The model under review builds one solid part; all positions refer to its coordinate system, in mm. Give positions to 0.01 mm unless a question says otherwise; leave off trailing zeros. Order: outer loops, then holes, each group sorted by start corner. A loop starts at its lowest first (then second) coordinate and runs counter-clockwise, first axis right, second up. Notation, with made-up numbers: (28.25, 77.25) - (32.25, 77.25) arc R16 cw to (32.25, 103.25) - close; hole circle Ø11 at (81, -40). An arc over 180 degrees is marked (long way). Use a Markdown table: item, result. Add a question column.
Autodesk Inventor part; units mm, degrees
ref_plane "YZ Plane" through (0, 0, 0) normal (1, 0, 0) x (0, 1, 0)
ref_plane "XZ Plane" through (0, 0, 0) normal (0, 1, 0) x (-1, 0, 0)
ref_plane "XY Plane" through (0, 0, 0) normal (0, 0, 1) x (1, 0, 0)
sketch "Sketch1" plane through (0, 0, 0) normal (0, 1, 0) x (-1, 0, 0)
  line L0 (169.8625, 0) -> (0, 0)
  line L1 (0, 0) -> (0, -169.8625)
  line L2 (0, -169.8625) -> (25.4, -169.8625)
  line L3 (25.4, -169.8625) -> (25.4, -103.8713)
  line L4 (103.8713, -25.4) -> (169.8625, -25.4)
  line L5 (169.8625, -25.4) -> (169.8625, 0)
  arc A0 (103.8713, -25.4) -> (25.4, -103.8713) centre (66.675, -66.675) ccw
  line L6 (0, 0) -> (66.675, -66.675) construction
  line L7 (0, -20) -> (6.35, -20)
  line L8 (6.35, -20) -> (6.35, -40)
  line L9 (6.35, -40) -> (0, -40)
  line L10 (0, -40) -> (0, -20)
  line L11 (6.35, -60) -> (6.35, -80)
  line L12 (0, -60) -> (6.35, -60)
  line L13 (6.35, -80) -> (0, -80)
  line L14 (6.35, -100) -> (6.35, -120)
  line L15 (0, -100) -> (6.35, -100)
  line L16 (6.35, -120) -> (0, -120)
  line L17 (6.35, -140) -> (6.35, -160)
  line L18 (0, -140) -> (6.35, -140)
  line L19 (6.35, -160) -> (0, -160)
  line L20 (23.368, -27.3469) -> (16.764, -27.3469)
  line L21 (16.764, -27.3469) -> (16.764, -12.0929)
  line L22 (16.764, -12.0929) -> (23.368, -12.0929)
  line L23 (23.368, -12.0929) -> (23.368, -27.3469)
  line L24 (23.368, -27.3469) -> (16.764, -12.0929) construction
  line L25 (16.764, -27.3469) -> (23.368, -12.0929) construction
  line L26 (25.4, -160) -> (16.764, -160)
  line L27 (16.764, -160) -> (16.764, -140)
  line L28 (16.764, -140) -> (25.4, -140)
  point P0 (103.8713, -25.4)
  point P1 (20.066, -19.7199)
  point P2 (20.066, -12.0929)
  dimension "d0" = 25.4
  dimension "d1" = 169.8625
  dimension "d2" = 25.4
  dimension "d3" = 169.8625
  dimension "d4" = 111.125
  dimension "d5" = 66.675
  dimension "d6" = 45
  dimension "d10" = 6.35
  dimension "d11" = 20
  dimension "d12" = 20
  dimension "d15" = 40
  dimension "d34" = 12.0929
  dimension "d35" = 6.604
  dimension "d36" = 20.066
  dimension "d37" = 15.254
extrude "Plate1" add sketch "Sketch1" along normal blind 7.9375 contours L5 L4 A0 L3 L28 L27 L26 L2 L1 L19 L17 L18 L16 L14 L15 L13 L11 L12 L9 L8 L7 L0
fillet "Corner Round1" radius 25.4 2 edges at (-103.8713, 3.9688, -25.4) (-25.4, 3.9688, -103.8713)
fillet "Corner Round2" radius 6 5 edges at (0, 3.9688, 0) (0, 3.9688, -169.8625) (-25.4, 3.9688, -169.8625) (-169.8625, 3.9688, 0) (-169.8625, 3.9688, -25.4)
sketch "Sketch2" plane through (0, 0, 0) normal (0, -1, 0) x (1, 0, 0)
  line L0 (-169.8625, -19.4) -> (-169.8625, -6)
  line L1 (-19.4, -169.8625) -> (-6, -169.8625)
  line L2 (-6, -169.8625) -> (-19.4, -169.8625)
  line L3 (0, -20) -> (0, -6)
  line L4 (-6, 0) -> (-163.8625, 0)
  point P0 (0, 0)
  point P1 (-165.1, -12.7)
  point P2 (-139.7, -12.7)
  point P3 (-114.3, -12.7)
  point P4 (-12.7, -165.1)
  point P5 (-12.7, -139.7)
  point P6 (-12.7, -114.3)
  point P7 (-169.8625, -12.7)
  point P8 (-169.8625, -12.7)
  point P9 (-12.7, -169.8625)
  point P10 (-12.7, -12.7)
  dimension "d21" = 25.4
  dimension "d22" = 25.4
  dimension "d23" = 25.4
  dimension "d24" = 25.4
  dimension "d25" = 4.7625
  dimension "d26" = 4.7625
  dimension "d38" = 12.7
  dimension "d39" = 12.7
hole "Hole1" at (-165.1, 0, -12.7) at (-139.7, 0, -12.7) at (-114.3, 0, -12.7) at (-12.7, 0, -165.1) at (-12.7, 0, -139.7) at (-12.7, 0, -114.3) at (-12.7, 0, -12.7) direction (0, 1, 0) diameter 5.105 depth 7.9375 tip angle 118
equation "\"d2\" = d0"
equation "\"d3\" = d1"
equation "\"d12\" = d11"
equation "\"d15\" = 2 * d11"
equation "\"d32\" = Thickness"
equation "\"d8\" = Thickness"
equation "\"BendRadius\" = Thickness"
equation "\"BendReliefWidth\" = Thickness"
equation "\"BendReliefDepth\" = 0.5 * Thickness"
equation "\"CornerReliefSize\" = 4 * Thickness"
equation "\"MinimumRemnant\" = 2 * Thickness"
equation "\"TransitionRadius\" = BendRadius"
equation "\"JacobiRadiusSize\" = BendRadius"
equation "\"GapSize\" = Thickness"
properties part number "INTAKE_SWERVE_MOUNT" material "Aluminum, 6061-T6"
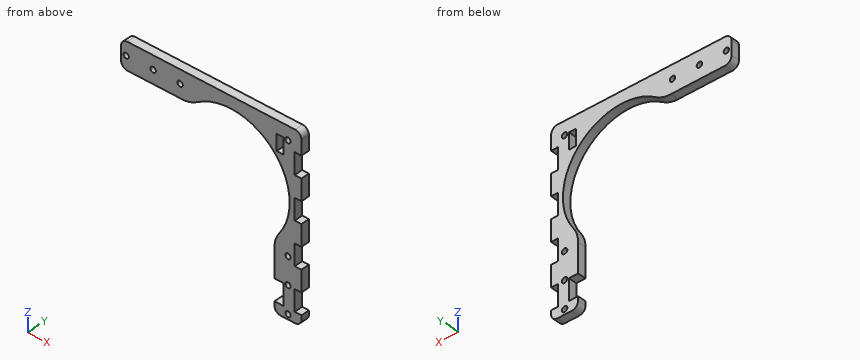
Q1. We need section B-B (y = 1.5). Count the separate pieces of the cut face and the enclosed holes in it, plus the area to 3 significant figures.
Q2. We need section A-A (x = -139.7). Write out the cut boundary in (y, z), plus the area to 3 significant figures.
Q3. Clearance check with flat-ended pins moving along their axes: P1, Ø4, axis at y = 7, z = -29.5, coming from the +X side; P2, Ø1.2, axis at y = 5, z = -162, coming from the -X side. State where each tip first meets the part, or that it passes through.
Q4. We need section D-D (x = -37.5). Write out the cut boundary in (y, z), plus the area to 3 significant figures.
Q5. We need section C-C (x = -78.5). Write out the cut boundary in (y, z), plus the area to 3 significant figures.
Q6. Wall thickness on probe 1 along X at (y, z) = (4.5, -114); probe 2 along Z at (x, y) = (-114.3, 2); probe 3 along Z at (x, y) = (-65, 6.25): over which ranges is each line inside the solid? List them lowest first.
Here are the results:
| question | item | result |
|---|---|---|
| 1 | separate pieces | 1 |
| 1 | enclosed holes | 8 |
| 1 | area | 5,560 mm2 |
| 2 | outline | (0, -25.4) - (7.94, -25.4) - (7.94, -15.25) - (0, -15.25) - close; (0, -10.15) - (7.94, -10.15) - (7.94, 0) - (0, 0) - close |
| 2 | area | 161 mm2 |
| 3 | P1 | x = -6.35 |
| 3 | P2 | x = -25.4 |
| 4 | outline | (0, -19.39) - (7.94, -19.39) - (7.94, 0) - (0, 0) - close |
| 4 | area | 154 mm2 |
| 5 | outline | (0, -12.39) - (7.94, -12.39) - (7.94, 0) - (0, 0) - close |
| 5 | area | 98.3 mm2 |
| 6 | probe 1 | -25.4 to -15.23, -10.17 to -6.35 |
| 6 | probe 2 | -25.4 to -15.25, -10.15 to 0 |
| 6 | probe 3 | -11.14 to 0 |
